Source: CAD feature listing. Evaluate the final solid. Frame: model axes, mm. Face numbers are marked on the shaded views. Coordinates: 2 decimals unless noted, no trailing zeros. Loops run counter-clockwise (first coordinate to the right, second up) from the corner with the lowest first, then second, coordinate; pieces in that order, holes last. Notation, with made-up numbers: (-6.75, 29.25) -> (14.25, 29.25) arc R23 cw to (14.25, 58.25) -> close; hole circle Ø6 at (60.5, 19). An arc over 180 degrees is marked (long way). Answer as CSV lines item,"result".
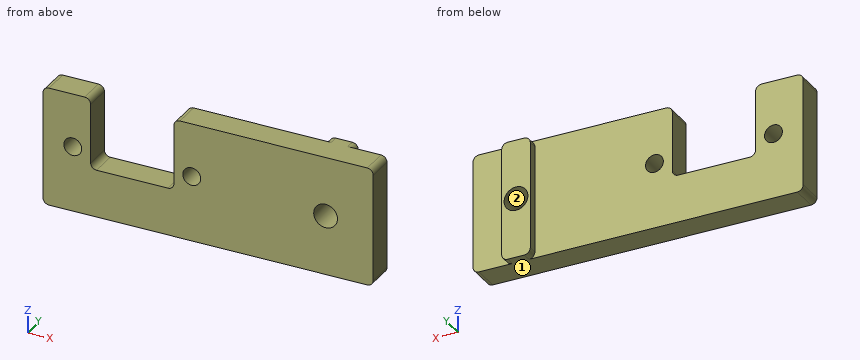
from build123d import *

# Parameters (mm, degrees)
ESQUISSE1_R             = 1.5
BOSS_EXTRU_1_DEPTH      = 4.5
CONG_1_R                = 1
ESQUISSE2_W             = 26.5
ESQUISSE2_H             = 20
BOSS_EXTRU_2_DEPTH      = 4.5
ESQUISSE3_W             = 4.8
ESQUISSE3_H             = 20
ESQUISSE3_R             = 2
BOSS_EXTRU_3_DEPTH      = 1.5
ESQUISSE4_R             = 2
ENL_V_MAT_EXTRU_1_DEPTH = 43.207819181
CONG_2_R                = 1


with BuildPart() as part:
    # Esquisse1 → Boss.-Extru.1 (new body)
    with BuildSketch(Plane(origin=(0, 0, 0), x_dir=(1, 0, 0), z_dir=(0, 1, 0))):
        Polygon((7, -9), (15, -9), (15, 11), (0, 11), (0, 3), (7, 3), align=None)
        with Locations(Location((10, 0, 0), (0, 0, 270))):
            Circle(ESQUISSE1_R, mode=Mode.SUBTRACT)
    extrude(amount=BOSS_EXTRU_1_DEPTH)

    # Congé1
    cong_1_edges = [part.edges().sort_by_distance(p)[0] for p in [
        (7, 2.25, -3),
        (15, 2.25, -11),
        (15, 2.25, 9),
        (7, 2.25, 9),
    ]]
    fillet(cong_1_edges, radius=CONG_1_R)

    # Symétrie1: part across plane


with BuildPart() as part_1:
    add(part.part)
    add(part.part.mirror(Plane(origin=(0, 4.5, -11), x_dir=(0, 0, 1), z_dir=(1, 0, 0))))

    # Esquisse2 → Boss.-Extru.2 (add)
    with BuildSketch(Plane(origin=(0, 4.5, 0), x_dir=(1, 0, 0), z_dir=(0, 1, 0))):
        with Locations((27.25, 1)):
            Rectangle(ESQUISSE2_W, ESQUISSE2_H)
    extrude(amount=-BOSS_EXTRU_2_DEPTH)

    # Esquisse3 → Boss.-Extru.3 (add)
    with BuildSketch(Plane.XZ.offset(-4.5)):
        with Locations((32.5, -1)):
            Rectangle(ESQUISSE3_W, ESQUISSE3_H)
        with Locations(Location((32.5, -1, 0), (0, 0, 270))):
            Circle(ESQUISSE3_R, mode=Mode.SUBTRACT)
    extrude(amount=-BOSS_EXTRU_3_DEPTH)

    # Esquisse4 → Enlèv. mat.-Extru.1 (cut, through all)
    with BuildSketch(Plane.XZ.offset(-4.5)):
        with Locations(Location((32.5, -1, 0), (0, 0, 270))):
            Circle(ESQUISSE4_R)
    extrude(amount=ENL_V_MAT_EXTRU_1_DEPTH, mode=Mode.SUBTRACT)

    # Congé2
    cong_2_edges = [part_1.edges().sort_by_distance(p)[0] for p in [
        (30.1, 5.25, 9),
        (30.1, 5.25, -11),
        (34.9, 5.25, -11),
        (34.9, 5.25, 9),
        (40.5, 2.25, -11),
        (40.5, 2.25, 9),
    ]]
    fillet(cong_2_edges, radius=CONG_2_R)


solid = part_1.part
(1) Cut plane C-C (y = 1.9). Return the cut outline in (x, z).
Computed values:
outline,"(-15, -10) arc R1 ccw to (-14, -11) -> (39.5, -11) arc R1 ccw to (40.5, -10) -> (40.5, 8) arc R1 ccw to (39.5, 9) -> (8, 9) arc R1 ccw to (7, 8) -> (7, -2) arc R1 cw to (6, -3) -> (-6, -3) arc R1 cw to (-7, -2) -> (-7, 8) arc R1 ccw to (-8, 9) -> (-14, 9) arc R1 ccw to (-15, 8) -> close; hole circle Ø3 at (-10, 0); hole circle Ø3 at (10, 0); hole circle Ø4 at (32.5, -1)"
(2) Cut plane A-A (z = 7.5). Return the cut outline in (x, y).
Computed values:
outline,"(-15, 0) -> (-7, 0) -> (-7, 4.5) -> (-15, 4.5) -> close; (7, 0) -> (40.5, 0) -> (40.5, 4.5) -> (34.9, 4.5) -> (34.9, 6) -> (30.1, 6) -> (30.1, 4.5) -> (7, 4.5) -> close"
(3) Material intervals for L1, parallel to X at y = 0.75, z = -0.5; L2, parallel to X at y = 4.05, z = -1; L3, parallel to Z at x = 32.5, y = 3.55, sorted ascending. Write a range as [from, to].
Computed values:
L1,"[-15, -11.41], [-8.59, -7], [7, 8.59], [11.41, 30.56], [34.44, 40.5]"
L2,"[-15, -11.12], [-8.88, -7], [7, 8.88], [11.12, 30.5], [34.5, 40.5]"
L3,"[-11, -3], [1, 9]"
(4) Cut plane D-D (z = -6.25). Return the cut outline in (x, y).
Computed values:
outline,"(-15, 0) -> (40.5, 0) -> (40.5, 4.5) -> (34.9, 4.5) -> (34.9, 6) -> (30.1, 6) -> (30.1, 4.5) -> (-15, 4.5) -> close"
(5) Pin query (flat end, axial travel): pin 1 Ø1.3 at (x, y) = (2.5, 3) entering from +Z; pin 2 Ø1.2 at (y, z) = (5.5, 2.5) entering from -X; pin 3 Ø2.5 at (x, z) = (10, 0) entering from -Y; pin 4 Ø4 at (x, z) = (-10, 0) entering from +Y. Return the tip coordinate at first contact, or that it passes through.
Computed values:
pin 1,"z = -3"
pin 2,"x = 30.1"
pin 3,"through"
pin 4,"y = 4.5"
(6) Cut plane B-B (x = 10). Return the cut outline in (y, z), then the cut area to 3 significant figures.
Computed values:
outline,"(0, -11) -> (4.5, -11) -> (4.5, -1.5) -> (0, -1.5) -> close; (0, 1.5) -> (4.5, 1.5) -> (4.5, 9) -> (0, 9) -> close"
area,"76.5 mm^2"
(7) Draft query along X for the marked faces 1 and 2. Return one class per face: released by +X, released by -X, zero draft, split by the parting line, or undercut.
Computed values:
face 1,"zero draft"
face 2,"undercut"
